Build history of the part. All positions in model axes, mm. Face numbers are marked on the shaded views. A direction names the side the tool comes from. Give positions to 0.01 mm unless a question says otherwise; leave off trailing zeros. Loops run counter-clockwise (first coordinate to the right, second up) from the corner with the lowest first, then second, coordinate; pieces in that order, holes last. Notation, with made-up numbers: (55, -38) -> (95, -38) arc R15 ccw to (95, -11) -> close; hole circle Ø9 at (-4, 48). An arc over 180 degrees is marked (long way). Answer as a JSON object with one key per item and string values. Group by question number.
Q1. Tool access for the marked faces 1, 2, 3, 4 and 5: list every direction of +Z, -Z, +X, -X, +Y, -Y with a clear straight run to the whole face (end or side of a thin tool).
Q2. Band-saw the part on C-C, the plane x = 24.5. Write the cut outline in (y, z).
Q3. Band-saw the part on D-D, the plane x = 17. Write the cut outline in (y, z), plus the area to 3 significant figures.
Q4. Drop flat-ended pins along their axis: pin 1 (3.5 mm diameter, centred on x = 16, z = 2, fed in from -Y); pin 2 (2.5 mm diameter, centred on y = -9, z = 1, fed in from -X); pin 3 (1.5 mm diameter, centred on x = 10.5, z = 2.5, fed in from +Y). Give the stop position or say it passes through.
Q5. Wall check: probe 1 along X at (y, z) = (-3.5, 1.5); probe 2 along Y at (x, z) = (28.5, 1.5); probe 3 along Z at (x, y) = (23.5, -0.5). Give the ranges that are in metal, low to high. Write a range as from..to.
Q6. Band-saw the part on A-A, the plane y = -11.25. Write the cut outline in (x, z), plus the area to 3 significant figures.
from build123d import *

# Parameters (mm, degrees)
EXTRUDE_1_DEPTH     = 3
SKETCH_1_3_R        = 2.25
EXTRUDE_2_DEPTH     = 10
SKETCH_2_W          = 5
SKETCH_2_H          = 2
CUT_EXTRUDE_1_DEPTH = 2
FILLET_1_R          = 4


with BuildPart() as part:
    # 草图1 → 凸台-拉伸1 (new body)
    with BuildSketch(Plane.XY):
        with BuildLine():
            Line((29.766666667, 3.993188645), (-0.13125, 2.246168613))
            ThreePointArc((-0.13125, 2.246168613), (-2.249041949, -0.065652955), (0, -2.25))
            Line((0, -2.25), (26, -2.25))
            Line((26, -2.25), (26, -20))
            Line((26, -20), (34, -20))
            Line((34, -20), (34, 0))
            ThreePointArc((34, 0), (32.744691847, 2.909753712), (29.766666667, 3.993188645))
        make_face()
        with BuildLine():
            Line((28.25, -16), (28.25, 0))
            ThreePointArc((28.25, 0), (30, 1.75), (31.75, 0))
            Line((31.75, 0), (31.75, -16))
            ThreePointArc((31.75, -16), (30, -17.75), (28.25, -16))
        make_face(mode=Mode.SUBTRACT)
    extrude(amount=EXTRUDE_1_DEPTH)

    # 草图1<3> → 凸台-拉伸2 (add)
    with BuildSketch(Plane.XY):
        with Locations(Location((0, 0, 0), (0, 0, 93.344152204))):
            Circle(SKETCH_1_3_R)
    extrude(amount=EXTRUDE_2_DEPTH)

    # 草图2 → 切除-拉伸1 (cut)
    with BuildSketch(Plane.XY.offset(10)):
        Rectangle(SKETCH_2_W, SKETCH_2_H)
    extrude(amount=-CUT_EXTRUDE_1_DEPTH, mode=Mode.SUBTRACT)

    # 圆角1
    fillet_1_edges = [part.edges().sort_by_distance(p)[0] for p in [
        (26, -20, 1.5),
        (34, -20, 1.5),
    ]]
    fillet(fillet_1_edges, radius=FILLET_1_R - 0.0001)  # a hair under: the kernel refuses the full size


solid = part.part
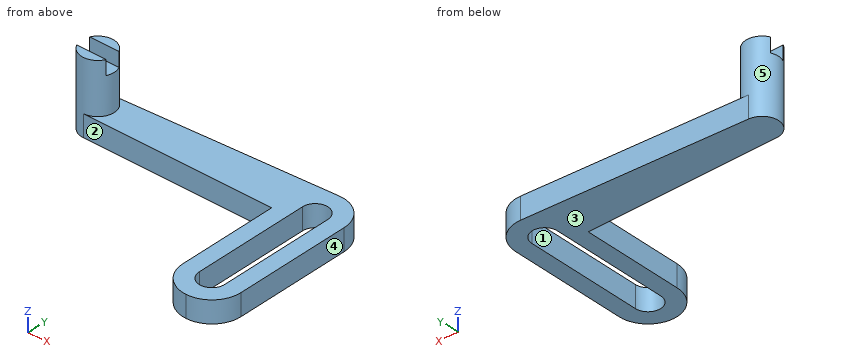
Worked answers:
{
 "1": {"face 1": "+Z, -Z", "face 2": "+Z, -Z, -X, -Y", "face 3": "-Z, +X, -X, +Y, -Y", "face 4": "+Z, -Z, +X, +Y, -Y", "face 5": "+Z"},
 "2": {"outline": "(-2.25, 0) -> (3.69, 0) -> (3.69, 3) -> (-2.25, 3) -> close"},
 "3": {"outline": "(-2.25, 0) -> (3.25, 0) -> (3.25, 3) -> (-2.25, 3) -> close", "area": "16.5 mm2"},
 "4": {"pin 1": "y = -2.25", "pin 2": "x = 26", "pin 3": "y = 2.91"},
 "5": {"probe 1": "26..28.25, 31.75..34", "probe 2": "-19.71..-16.9, 0.9..3.92", "probe 3": "0..3"},
 "6": {"outline": "(26, 0) -> (28.25, 0) -> (28.25, 3) -> (26, 3) -> close; (31.75, 0) -> (34, 0) -> (34, 3) -> (31.75, 3) -> close", "area": "13.5 mm2"}
}
